Geometry: final body of the model. Coordinates: model frame, mm. Face numbers are marked on the shaded views. Give positions to 0.01 mm unless a question says otherwise; leave off trailing zeros. Loops run counter-clockwise (first coordinate to the right, second up) from the corner with the lowest first, then second, coordinate; pieces in that order, holes last. Notation, with made-up numbers: (48, -40) - (91, -40) arc R24 ccw to (91, -13) - close; hole circle Ø4 at (31, 48). An arc over 180 degrees is marked (long way). Use one line per item in the form item = value.
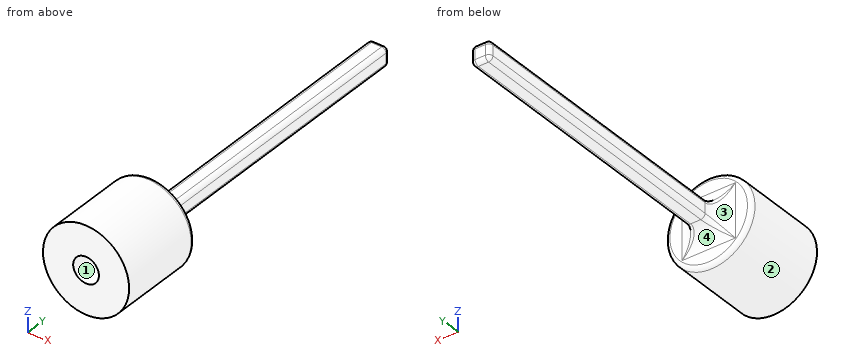
```python
from build123d import *

# Parameters (mm, degrees)
SKETCH1_R                  = 6.35
BOSS_EXTRUDE1_DEPTH        = 12.7
SKETCH2_W                  = 2.778125
SKETCH2_H                  = 2.778125
BOSS_EXTRUDE2_DEPTH        = 44.45
FILLET1_R                  = 2.54
FILLET2_R                  = 0.635
F_10_24_TAPPED_HOLE1_D     = 3.7973
F_10_24_TAPPED_HOLE1_DEPTH = 9.525
F_10_24_TAPPED_HOLE1_TIP   = 1.140824014


with BuildPart() as part:
    # Sketch1 → Boss-Extrude1 (new body)
    with BuildSketch(Plane(origin=(0, 0, 0), x_dir=(0, 0, -1), z_dir=(0, 1, 0))):
        with Locations(Location((0, 0, 0), (0, 0, 180))):
            Circle(SKETCH1_R)
    extrude(amount=BOSS_EXTRUDE1_DEPTH)

    # Sketch2 → Boss-Extrude2 (add)
    with BuildSketch(Plane(origin=(-12.7, 12.7, 0), x_dir=(0, 0, -1), z_dir=(0, -1, 0))):
        with Locations((0, 12.7)):
            Rectangle(SKETCH2_W, SKETCH2_H)
    extrude(amount=-BOSS_EXTRUDE2_DEPTH)

    # Fillet1
    fillet1_edges = [part.edges().sort_by_distance(p)[0] for p in [
        (0, 12.7, -1.3890625),
        (-1.3890625, 12.7, 0),
        (1.3890625, 12.7, 0),
        (0, 12.7, 1.3890625),
    ]]
    fillet(fillet1_edges, radius=FILLET1_R)

    # Fillet2
    fillet2_edges = [part.edges().sort_by_distance(p)[0] for p in [
        (2.288098275, 13.301228117, -2.288098275),
        (-2.288098218, 13.301228166, -2.288098218),
        (2.288098215, 13.301228168, 2.288098215),
        (-2.288098198, 13.301228182, 2.288098198),
        (0, 12.7, -6.35),
        (1.3890625, 36.195, -1.3890625),
        (-1.3890625, 36.195, -1.3890625),
        (0, 57.15, 1.3890625),
        (-1.3890625, 36.195, 1.3890625),
        (1.3890625, 57.15, 0),
        (1.3890625, 36.195, 1.3890625),
        (0, 57.15, -1.3890625),
        (-1.3890625, 57.15, 0),
    ]]
    fillet(fillet2_edges, radius=FILLET2_R)

    # #10-24 Tapped Hole1
    with Locations(Plane(origin=(0, 0, 0), x_dir=(-1, 0, 0), z_dir=(0, -1, 0))):
        with Locations((0, 0)):
            Hole(F_10_24_TAPPED_HOLE1_D / 2, depth=F_10_24_TAPPED_HOLE1_DEPTH)
            with Locations((0, 0, -(F_10_24_TAPPED_HOLE1_DEPTH + F_10_24_TAPPED_HOLE1_TIP / 2))):  # 118° drill point
                Cone(0, F_10_24_TAPPED_HOLE1_D / 2, F_10_24_TAPPED_HOLE1_TIP, mode=Mode.SUBTRACT)


solid = part.part
```
(1) Cut plane B-B (y = 8). Return the cut outline in (x, z).
Solution:
outline = circle Ø12.7 at (0, 0); hole circle Ø3.8 at (0, 0)
(2) Pin query (flat end, axial travel): P1, Ø0.5, axis at x = 0, y = 37.5, coming from the +Z side; P2, Ø0.5, axis at y = 39.5, z = 0, coming from the -X side; P3, Ø1.7, axis at y = 31.5, z = -0.5, coming from the +X side. Return the tip coordinate at first contact, or that it passes through.
Solution:
P1 = 1.39
P2 = -1.39
P3 = 1.39
(3) Material intervals for L1, parallel to Z at x = 0.25, y = 37; L2, parallel to Z at x = -1, y = 7, sorted ascending. Write a range as from..to.
Solution:
L1 = -1.39..1.39
L2 = -6.27..-1.61, 1.61..6.27
(4) Pull-direction query (X, two-part tool) for the marked faces 1, 2, 3 and 4; classes: released by +X, released by -X, zero draft, split by the parting line, or undercut.
Solution:
face_1 = undercut
face_2 = split by the parting line
face_3 = released by -X
face_4 = zero draft
(5) Cut plane A-A (y = 43). Return the cut outline in (x, z) (3 decimals), plus the area to 3 significant figures.
Solution:
outline = (-1.389, -0.754) arc R0.635 ccw to (-0.754, -1.389) - (0.754, -1.389) arc R0.635 ccw to (1.389, -0.754) - (1.389, 0.754) arc R0.635 ccw to (0.754, 1.389) - (-0.754, 1.389) arc R0.635 ccw to (-1.389, 0.754) - close
area = 7.37 mm2
